Work out the finished part from the listing and answer in its coordinate system (mm). Coordinates: 2 decimals unless noted, no trailing zeros. Order: outer loops, then holes, each group sorted by start corner. A loop starts at its lowest first (then second) coordinate and runs counter-clockwise, first axis right, second up. Notation, with made-up numbers: (75, 8) - (106, 8) arc R16 cw to (106, 22) - close; hole circle Ø1 at (74.5, -34). An arc over 180 degrees is marked (long way). Answer as a JSON object with one key per item and string values. Group by question number.
1) Each of these flat-tipped pins is pushed along its axis until it touches: P1, Ø3, axis at x = 67.5, y = 2, coming from the -Z side; P2, Ø1.9, axis at x = 30, y = -1, coming from the +Z side; P3, Ø1.9, axis at y = -1, z = 36, coming from the -X side. Where does it stop, or does it pass through?
2) Section A-A (z = -19) is taken. Give the vertices of the cut face in (x, y) (3 decimals), plus the area to 3 significant figures.
3) Section B-B (y = -1) is taken. Give the vertices of the cut face in (x, z), plus the area to 3 significant figures.
4) Section C-C (x = -27.5) is taken. Give the vertices of the cut face in (y, z) (3 decimals).
5) Find the intervals of material crossed by line 1 along X through (y, z) = (0.25, 1.5); line 2 along Z through (x, y) = (55, -1.25), in increasing order.
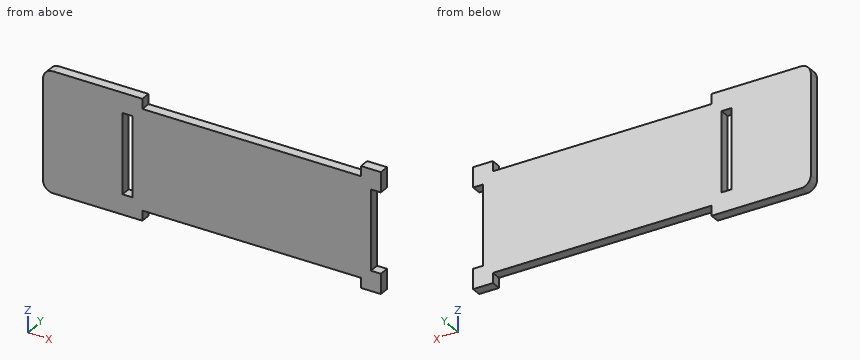
from build123d import *

# Parameters (mm, degrees)
SKETCH1_W           = 6.35
SKETCH1_H           = 50.8
BOSS_EXTRUDE1_DEPTH = 3.175


with BuildPart() as part:
    # Sketch1 → Boss-Extrude1 (new, symmetric)
    with BuildSketch(Plane(origin=(0, 0, 0), x_dir=(1, 0, 0), z_dir=(0, 1, 0))):
        with BuildLine():
            Line((-101.6, -38.1), (-44.45, -38.1))
            Line((-44.45, -38.1), (-44.45, -31.75))
            Line((-44.45, -31.75), (95.25, -31.75))
            Line((95.25, -31.75), (95.25, -38.1))
            Line((95.25, -38.1), (107.95, -38.1))
            Line((107.95, -38.1), (107.95, -25.4))
            Line((107.95, -25.4), (101.6, -25.4))
            Line((101.6, -25.4), (101.6, 25.4))
            Line((101.6, 25.4), (107.95, 25.4))
            Line((107.95, 25.4), (107.95, 38.1))
            Line((107.95, 38.1), (95.25, 38.1))
            Line((95.25, 38.1), (95.25, 31.75))
            Line((95.25, 31.75), (-44.45, 31.75))
            Line((-44.45, 31.75), (-44.45, 38.1))
            Line((-44.45, 38.1), (-101.6, 38.1))
            ThreePointArc((-101.6, 38.1), (-106.090128061, 36.240128061), (-107.95, 31.75))
            Line((-107.95, 31.75), (-107.95, -31.75))
            ThreePointArc((-107.95, -31.75), (-106.090128061, -36.240128061), (-101.6, -38.1))
        make_face()
        with Locations((-53.975, 0)):
            Rectangle(SKETCH1_W, SKETCH1_H, mode=Mode.SUBTRACT)
    extrude(amount=BOSS_EXTRUDE1_DEPTH, both=True)


solid = part.part
Report:
{
 "1": {"P1": "stops at z = -31.75", "P2": "stops at z = 31.75", "P3": "stops at x = -107.03"},
 "2": {"outline": "(-107.95, -3.175) - (-57.15, -3.175) - (-57.15, 3.175) - (-107.95, 3.175) - close; (-50.8, -3.175) - (101.6, -3.175) - (101.6, 3.175) - (-50.8, 3.175) - close", "area": "1,290 mm²"},
 "3": {"outline": "(-107.95, -31.75) arc R6.35 ccw to (-101.6, -38.1) - (-44.45, -38.1) - (-44.45, -31.75) - (95.25, -31.75) - (95.25, -38.1) - (107.95, -38.1) - (107.95, -25.4) - (101.6, -25.4) - (101.6, 25.4) - (107.95, 25.4) - (107.95, 38.1) - (95.25, 38.1) - (95.25, 31.75) - (-44.45, 31.75) - (-44.45, 38.1) - (-101.6, 38.1) arc R6.35 ccw to (-107.95, 31.75) - close; hole (-57.15, -25.4) - (-50.8, -25.4) - (-50.8, 25.4) - (-57.15, 25.4) - close", "area": "14,000 mm²"},
 "4": {"outline": "(-3.175, -31.75) - (3.175, -31.75) - (3.175, 31.75) - (-3.175, 31.75) - close"},
 "5": {"line 1": "x = -107.95 to -57.15, -50.8 to 101.6", "line 2": "z = -31.75 to 31.75"}
}
